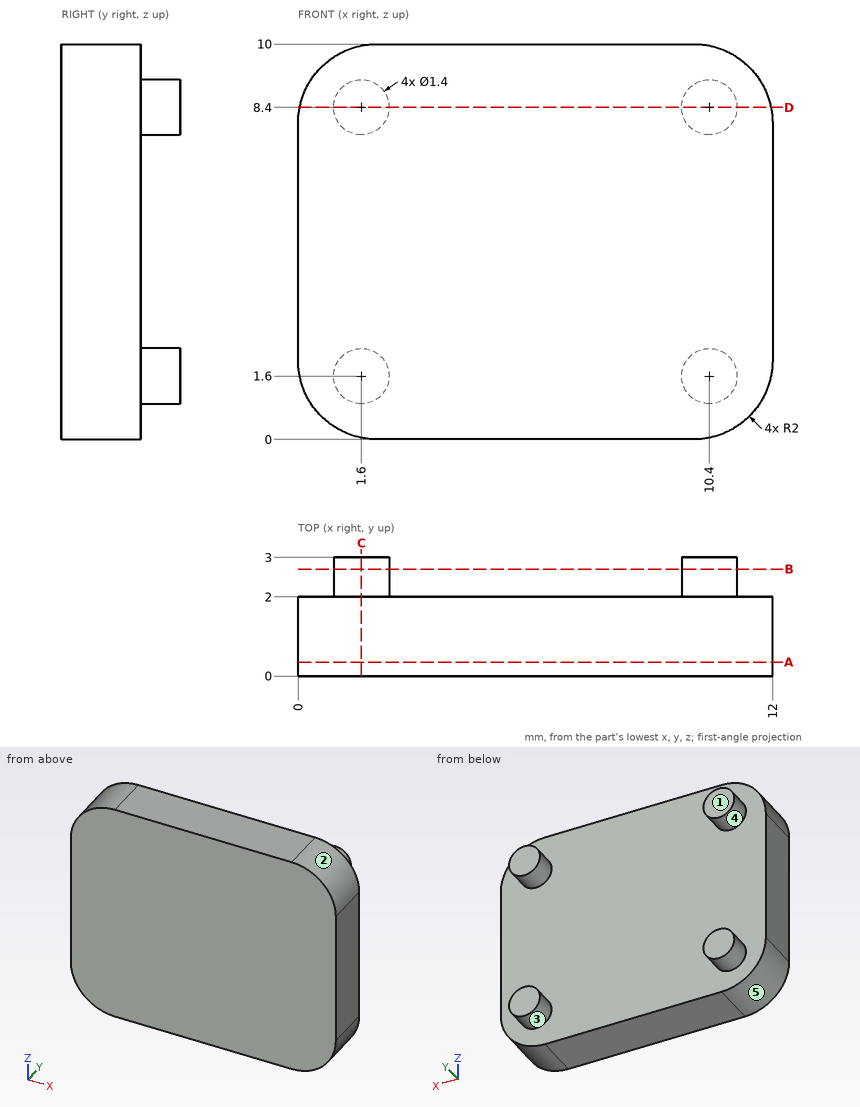
Input: dimensioned drawing with shaded views. Units: mm. Origin: part minimum x, y, z. A direction names the side the tool comes from. Give positions to 0.01 mm unless a question says otherwise; leave off trailing zeros. Order: outer loops, then holes, each group sorted by start corner. A loop starts at its lowest first (then second) coordinate and runs counter-clockwise, first axis right, second up. Notation, with made-up numbers: (64.25, 85.5) -> (118.25, 85.5) arc R27 cw to (118.25, 114.5) -> close; hole circle Ø8 at (-16.75, 46.5). An arc over 180 degrees is marked (long way). Use one line per item in the form item = value.
1) Section C-C, the plane x = 1.6. Return loops of the section in (y, z), and give its area (3 significant figures).
Response values:
outline = (0, 0.04) -> (2, 0.04) -> (2, 0.9) -> (3, 0.9) -> (3, 2.3) -> (2, 2.3) -> (2, 7.7) -> (3, 7.7) -> (3, 9.1) -> (2, 9.1) -> (2, 9.96) -> (0, 9.96) -> close
area = 22.6 mm^2
2) Reachability of the marked faces 4 and 5 from +Z, -Z, +X, -X, +Y, -Y: full face, straight path, thin tool, end or side. Return the list, or none.
Response values:
face_4 = +Y
face_5 = -Z, -X, +Y, -Y
3) Section A-A, the plane y = 0.35. Return loops of the section in (x, z), and give its area (3 significant figures).
Response values:
outline = (0, 2) arc R2 ccw to (2, 0) -> (10, 0) arc R2 ccw to (12, 2) -> (12, 8) arc R2 ccw to (10, 10) -> (2, 10) arc R2 ccw to (0, 8) -> close
area = 117 mm^2
4) Section D-D, the plane z = 8.4. Return loops of the section in (x, y).
Response values:
outline = (0.04, 0) -> (11.96, 0) -> (11.96, 2) -> (11.1, 2) -> (11.1, 3) -> (9.7, 3) -> (9.7, 2) -> (2.3, 2) -> (2.3, 3) -> (0.9, 3) -> (0.9, 2) -> (0.04, 2) -> close
5) Mould query, pull axis Z, two halves, no side actions, for the marked faces 1, 2 and 3. Classes: pulls with the +Z half, pulls with the -Z half, needs draft (parallel to the pull), parting line crosses it, or undercut.
Response values:
face_1 = needs draft
face_2 = pulls with the +Z half
face_3 = undercut
6) Line query: probe 1 along Y at (x, z) = (8, 4); probe 2 along Z at (x, y) = (11, 0.4); probe 3 along X at (y, z) = (1.55, 1). Output: solid intervals per line, ascending.
Response values:
probe_1 = 0 to 2
probe_2 = 0.27 to 9.73
probe_3 = 0.27 to 11.73
7) Section B-B, the plane y = 2.7. Return loops of the section in (x, z).
Response values:
outline = circle Ø1.4 at (1.6, 1.6); circle Ø1.4 at (1.6, 8.4); circle Ø1.4 at (10.4, 1.6); circle Ø1.4 at (10.4, 8.4)
